CAD build for the part. Positions are in the model's coordinates, mm. A direction names the side the tool comes from. Round coordinates to 2 decimals unless told otherwise and drop trailing zeros. Loops run counter-clockwise (first coordinate to the right, second up) from the corner with the lowest first, then second, coordinate; pieces in that order, holes last.
from build123d import *

# Parameters (mm, degrees)
EXTRUDE_1_DEPTH          = 12.75
EXTRUDE_1_DEPTH_BACK     = 12.75
EXTRUDE_1_2_DEPTH        = 1.2
EXTRUDE_2_DEPTH          = 1.2
SKETCH_4_W               = 23.6
SKETCH_4_H               = 23.6
CUT_EXTRUDE_1_DEPTH      = 1.5
CUT_EXTRUDE_2_DEPTH      = 35.680906203
CUT_EXTRUDE_2_DEPTH_BACK = 35.680906203
SKETCH_5_W               = 13.95
SKETCH_5_H               = 32.801494515


with BuildPart() as part:
    # Эскиз1 → Extrude 1 (new, two sides: drawn at the far end of the back side and taken through both)
    with BuildSketch(Plane.XY.offset(-EXTRUDE_1_DEPTH_BACK)):
        Polygon((-17.621320344, -13.5), (17.621320344, -13.5), (25.211407429, -5.909912914), (0, 19.301494515), (-25.211407429, -5.909912914), align=None)
        Polygon((-17, -12), (17, -12), (23.090087086, -5.909912914), (0, 17.180174171), (-23.090087086, -5.909912914), align=None, mode=Mode.SUBTRACT)
    extrude(amount=EXTRUDE_1_DEPTH + EXTRUDE_1_DEPTH_BACK)

    # Эскиз2 → Extrude 1 2 (add)
    with BuildSketch(Plane.XY.offset(12.75)):
        Polygon((25.211407429, -5.909912914), (0, 19.301494515), (-25.211407429, -5.909912914), (-17.621320344, -13.5), (17.621320344, -13.5), align=None)
    extrude(amount=EXTRUDE_1_2_DEPTH)

    # Эскиз3 → Бобышка-Вытянуть2 (add)
    with BuildSketch(Plane(origin=(0, 0, -12.75), x_dir=(-1, 0, 0), z_dir=(0, 0, -1))):
        Polygon((0, 19.301494515), (25.211407429, -5.909912914), (17.621320344, -13.5), (-17.621320344, -13.5), (-25.211407429, -5.909912914), align=None)
    extrude(amount=EXTRUDE_2_DEPTH)

    # Эскиз4 → Вырез-Вытянуть1 (cut)
    with BuildSketch(Plane.XZ.offset(13.5)):
        Rectangle(SKETCH_4_W, SKETCH_4_H)
    extrude(amount=-CUT_EXTRUDE_1_DEPTH, mode=Mode.SUBTRACT)

    # Эскиз5 → Вырез-Вытянуть2 (cut, two sides: drawn at the far end of the back side and taken through both)
    with BuildSketch(Plane(origin=(0, 0, 0), x_dir=(0, 0, -1), z_dir=(1, 0, 0)).offset(-CUT_EXTRUDE_2_DEPTH_BACK)):
        with Locations((6.975, 2.900747258)):
            Rectangle(SKETCH_5_W, SKETCH_5_H)
    extrude(amount=CUT_EXTRUDE_2_DEPTH + CUT_EXTRUDE_2_DEPTH_BACK, mode=Mode.SUBTRACT)


solid = part.part
Item 1: Mould opens along Y. For faces 4 (the flat face through (-11.38, 5.8, 6.29)), 5 (the flat face through (-4, -13.5, 13)), 6 (the flat face through (12.8, 6.5, 7.1)) say: released by +Y, released by -Y, zero draft, split by the parting line, or undercut.
Verdict:
face 4: undercut
face 5: released by -Y
face 6: released by +Y
Item 2: Wall check: L1, parallel to Z at x = 10.5, y = -5; L2, parallel to X at y = 10.5, z = 6; L3, parallel to X at y = 11.5, z = 10.25. Give the ranges that are in metal, low to high.
Verdict:
L1: z = 12.75 to 13.95
L2: x = -8.8 to -6.68, 6.68 to 8.8
L3: x = -7.8 to -5.68, 5.68 to 7.8
Item 3: Flat gauge pins, fed straight in: P1, Ø8, axis at y = 10.5, z = 10.5, coming from the +X side; P2, Ø1, axis at y = 4.5, z = 8, coming from the +X side; P3, Ø0.8, axis at y = -13, z = 5.5, coming from the -X side. Where does each tip first touch, or does it go through?
Verdict:
P1: stops at x = 12.8
P2: stops at x = 15.3
P3: stops at x = -18.52
Item 4: Cut at B-B (x = 14). List the corners of the cut face in (y, z), plus the area to 3 significant figures.
Verdict:
outline: (-13.5, 0) - (-12, 0) - (-12, 12.75) - (3.18, 12.75) - (3.18, 0) - (5.3, 0) - (5.3, 13.95) - (-13.5, 13.95) - close
area: 68.7 mm2
Item 5: Cut at C-C (y = 12.5). List the corners of the cut face in (x, z).
Verdict:
outline: (-6.8, 0) - (-4.68, 0) - (-4.68, 12.75) - (4.68, 12.75) - (4.68, 0) - (6.8, 0) - (6.8, 13.95) - (-6.8, 13.95) - close
Item 6: Cut at A-A (z = 2.25). List the corners of the cut face in (x, y), plus the area to 3 significant figures.
Verdict:
outline: (-25.21, -5.91) - (-17.62, -13.5) - (-11.8, -13.5) - (-11.8, -12) - (-17, -12) - (-23.09, -5.91) - (0, 17.18) - (23.09, -5.91) - (17, -12) - (11.8, -12) - (11.8, -13.5) - (17.62, -13.5) - (25.21, -5.91) - (0, 19.3) - close
area: 148 mm2
Item 7: 3-axis set-ups, long thin cutter, end or side, ignore diameter. For faces 1 (the flat face through (11.71, 5.47, 6.29)), 2 (the flat face through (0, -13, 11.8)), 3 (the flat face through (7.4, 10.1, 0)): which of +Z, -Z, +X, -X, +Y, -Y reach the whole face in a straight line?
Verdict:
face 1: -Z
face 2: -Z, -Y
face 3: -Z, +X, -X, +Y, -Y
